from build123d import *

# Parameters (mm, degrees)
SALIENTE_EXTRUIR1_DEPTH = 3
CORTAR_EXTRUIR1_DEPTH   = 10


with BuildPart() as part:
    # Croquis1 → Saliente-Extruir1 (new body)
    with BuildSketch(Plane(origin=(0, 0, 0), x_dir=(1, 0, 0), z_dir=(0, 1, 0))):
        Polygon((3, 35.5), (0, 35.5), (0, 47.5), (3, 47.5), (3, 59.5), (0, 59.5), (0, 71.5), (3, 71.5), (3, 80), (13.5, 80), (13.5, 83), (47.5, 83), (47.5, 80), (61, 80), (61, 71.5), (58, 71.5), (58, 59.5), (61, 59.5), (61, 47.5), (58, 47.5), (58, 35.5), (61, 35.5), (61, 23.5), (58, 23.5), (58, 11.5), (61, 11.5), (61, 3), (47.5, 3), (47.5, 0), (13.5, 0), (13.5, 3), (3, 3), (3, 11.5), (0, 11.5), (0, 23.5), (3, 23.5), align=None)
    extrude(amount=SALIENTE_EXTRUIR1_DEPTH)

    # Croquis2 → Cortar-Extruir1 (cut)
    with BuildSketch(Plane(origin=(0, 3, 0), x_dir=(1, 0, 0), z_dir=(0, 1, 0))):
        Polygon((15.5, 41.5), (15.5, 45.5), (12.5, 45.5), (12.5, 37.5), (15.5, 37.5), align=None)
        Polygon((45.5, 37.5), (45.5, 41.5), (45.5, 45.5), (48.5, 45.5), (48.5, 37.5), align=None)
    extrude(amount=-CORTAR_EXTRUIR1_DEPTH, mode=Mode.SUBTRACT)


solid = part.part
Work out the finished part from the listing and answer in its coordinate system (mm). A direction names the side the tool comes from. Coordinates: 2 decimals unless noted, no trailing zeros. Write each loop counter-clockwise with the first axis right and the second up, starting at its lowest first coordinate (ties: lowest second). Pieces come first, ordered by that corner, then holes. Notation, with made-up numbers: M -21,-37.5 L 23,-37.5 A11 ccw 23,-18.5 Z; hole C 28,4.5 d9. An arc over 180 degrees is marked long. Use one line per item in the form item = value. Start each with the question number.
1. The part is cut by section D-D (z = -32.5). Give the vertices of the cut face in (x, y).
2. The part is cut by section C-C (x = 57). Give the vertices of the cut face in (y, z), plus the area to 3 significant figures.
3. Each of these flat-tipped pins is pushed along its axis until it touches: P1, Ø1.5, axis at x = 54.5, y = 1.5, coming from the +Z side; P2, Ø1.5, axis at x = 59.5, y = 1, coming from the -Z side; P3, Ø1.5, axis at y = 2, z = -75.5, coming from the -X side. Where does it stop, or does it pass through?
4. The mould has two halves that part along Z. Classify faces 5 (the face through (31, 1, 0)), 6 (the face through (1, 1, -71.5)), 7 (the face through (60, 1, -23.5)), 8 (the face through (0, 1, -41)): released by +Z, released by -Z, zero draft, split by the parting line, or undercut.
5. A tool of negligible diameter and unlimited length cuts with its end or side. For faces 1 (the face through (58, 1, -66)), 2 (the face through (45.5, 2, -42)), 3 (the face through (13.5, 1, -1)), 4 (the face through (13.5, 1, -81)), from which of +Z, -Z, +X, -X, +Y, -Y can it reach the whole face along a straight path? Write none if from no direction.
6. The part is cut by section B-B (y = 2.4). Give the number of separate pieces and of enclosed holes in the cut face, plus the area to 3 significant figures.
7. Straight lines are drawn through the part: probe 1 along X at (y, z) = (1.4, -39); probe 2 along Z at (x, y) = (14, 2); probe 3 along Z at (x, y) = (7, 0.4). For each, find the intervals that lie inside material, in ascending order. Write a range as from..to.
8. The part is cut by section A-A (z = -41.5). Give the vertices of the cut face in (x, y), plus the area to 3 significant figures.
Evaluation:
q1.outline = M 3,0 L 61,0 L 61,3 L 3,3 Z
q2.outline = M 0,-80 L 3,-80 L 3,-3 L 0,-3 Z
q2.area = 231 mm^2
q3.P1 = -3
q3.P2 = -80
q3.P3 = 3
q4.face_5 = released by +Z
q4.face_6 = released by -Z
q4.face_7 = undercut
q4.face_8 = zero draft
q5.face_1 = +X, +Y, -Y
q5.face_2 = +Y, -Y
q5.face_3 = +Z, -X, +Y, -Y
q5.face_4 = -Z, -X, +Y, -Y
q6.separate_pieces = 1
q6.enclosed_holes = 2
q6.area = 4,620 mm^2
q7.probe_1 = 0..12.5, 15.5..45.5, 48.5..58
q7.probe_2 = -83..-45.5, -37.5..0
q7.probe_3 = -80..-3
q8.outline = M 0,0 L 12.5,0 L 12.5,3 L 0,3 Z; M 15.5,0 L 45.5,0 L 45.5,3 L 15.5,3 Z; M 48.5,0 L 58,0 L 58,3 L 48.5,3 Z
q8.area = 156 mm^2
